Could you check a few things on this model? Use its own coordinates, in mm. A direction names the side the tool comes from. Round coordinates to 2 decimals unless told otherwise and drop trailing zeros. Write each loop counter-clockwise with the first axis right and the second up, starting at its lowest first coordinate (ties: lowest second). Pieces come first, ordered by that corner, then holes. Notation, with made-up numbers: M -28,20.5 L 8,20.5 A15 ccw 8,36.5 Z; hole C 44.25,70 d7. An arc over 180 degrees is marked long. One line per item, written item: value. Start each with the question number.
(1) I want a section at D-D on z = 0.5. Please give me the cut outline in (x, y), and give its area (4 significant figures).
(2) I want a section at C-C on x = -1. Please give me the cut outline in (y, z).
(3) I want a section at B-B on z = 5. Please give me the cut outline in (x, y).
(4) Which directions (+Z, -Z, +X, -X, +Y, -Y) give clear straight access to the entire face, cutting with the end or side of a thin tool? Please do faces 5 (the face through (-12, -12, 6)), 6 (the face through (5, 6, 1)), 7 (the face through (-9, -11, 4)).
(5) I want a section at A-A on y = -5.25. Please give me the cut outline in (x, z).
(6) Thinking about a two-plate mould opening in Z: for faces 1 (the face through (12, -12, 6)), 2 (the face through (-10, -13, 3)), 3 (the face through (-9.36, 11.99, 5.84)), 4 (the face through (8.9, -12, 5)), which applies, released by +Z, released by -Z, zero draft, split by the parting line, or undercut?
(7) I'm going to push flat-ended pins straight in: pin 1 Ø3 at (x, y) = (-5.5, 5) entering from +Z; pin 2 Ø2 at (x, z) = (-4.5, 2) entering from -Y; pin 3 Ø2.5 at (x, z) = (-2.5, 6) entering from -Y. Where does each tip first touch, or does it pass through?
(8) If I drill on L1, parallel to Y at x = 4.75, z = 1.75; L2, parallel to Z at x = -9.9, y = -11.7; L3, parallel to Y at x = 2, z = 5.5, over which ranges is the centre line in solid material (lowest first)?
```python
from build123d import *

# Parameters (mm, degrees)
F0_W        = 26
F0_H        = 2
F1_DEPTH    = 8
F0_W_2      = 6.25
F2_DEPTH    = 3
F3_T1_DEPTH = 27
F3_T3_DEPTH = 27
F4_R        = 1
F5_DEPTH    = 30


# Not quite as in the source:
# - a fillet or chamfer that OpenCascade refuses, or shapes differently, is made with other operations: its cross-section is extruded or revolved along the edge and cut away or added


with BuildPart() as f1:
    # F0 (on Top) → F1 (new body)
    with BuildSketch(Plane.XY):
        with Locations((0, 12)):
            Rectangle(F0_W, F0_H)
    extrude(amount=F1_DEPTH)



with BuildPart() as f1b:
    # F0 (on Top) → F1, piece 2 (new body)
    with BuildSketch(Plane.XY):
        with Locations((-9.875, -12)):
            Rectangle(F0_W_2, F0_H)
    extrude(amount=F1_DEPTH)


with BuildPart() as f1c:
    # F0 (on Top) → F1, piece 3 (new body)
    with BuildSketch(Plane.XY):
        with Locations((9.875, -12)):
            Rectangle(F0_W_2, F0_H)
    extrude(amount=F1_DEPTH)


with BuildPart() as f1_1:
    add(f1.part)

    add(f1b.part)  # F2 merges F1b

    add(f1c.part)  # F2 merges F1c
    # F0 (on Top) → F2 (join)
    with BuildSketch(Plane.XY):
        Polygon((6.75, -11), (13, -11), (13, 11), (-13, 11), (-13, -11), (-6.75, -11), (-6.75, 6), (-3.9725974202, 6), (-3.9725974202, 7), (4.0274025798, 7), (4.0274025798, 6), (6.75, 6), align=None)
    extrude(amount=F2_DEPTH)

    # F3: fillet of radius 5 on 6 edges, made by hand

    # F3_s2 → F3_t1 (cut)
    with BuildSketch(Plane.XZ.offset(-1.5)):
        with BuildLine():
            ThreePointArc((-8, 8), (-11.5355339059, 6.5355339059), (-13, 3))
            Line((-13, 3), (-13, 8))
            Line((-13, 8), (-8, 8))
        make_face()
        with BuildLine():
            ThreePointArc((-6.75, 3), (-8.2144660941, 6.5355339059), (-11.75, 8))
            Line((-11.75, 8), (-6.75, 8))
            Line((-6.75, 8), (-6.75, 3))
        make_face()
        with BuildLine():
            ThreePointArc((11.75, 8), (8.2144660941, 6.5355339059), (6.75, 3))
            Line((6.75, 3), (6.75, 8))
            Line((6.75, 8), (11.75, 8))
        make_face()
        with BuildLine():
            ThreePointArc((8, 8), (11.5355339059, 6.5355339059), (13, 3))
            Line((13, 3), (13, 8))
            Line((13, 8), (8, 8))
        make_face()
    extrude(amount=F3_T1_DEPTH, mode=Mode.SUBTRACT)

    # F3_s4 → F3_t3 (cut)
    with BuildSketch(Plane.XZ.offset(-25.5)):
        with BuildLine():
            ThreePointArc((8, 8), (11.5355339059, 6.5355339059), (13, 3))
            Line((13, 3), (13, 8))
            Line((13, 8), (8, 8))
        make_face()
        with BuildLine():
            ThreePointArc((-13, 3), (-11.5355339059, 6.5355339059), (-8, 8))
            Line((-8, 8), (-13, 8))
            Line((-13, 8), (-13, 3))
        make_face()
    extrude(amount=F3_T3_DEPTH, mode=Mode.SUBTRACT)

    # F4 (on face) → F5 (cut)
    with BuildSketch(Plane.XZ.offset(13)):
        with Locations((-9.9, 5)):
            Circle(F4_R)
        with Locations((9.9, 5)):
            Circle(F4_R)
    extrude(amount=-F5_DEPTH, mode=Mode.SUBTRACT)


solid = f1_1.part
```
Found:
1. outline: M -13,-13 L -6.75,-13 L -6.75,6 L -3.97,6 L -3.97,7 L 4.03,7 L 4.03,6 L 6.75,6 L 6.75,-13 L 13,-13 L 13,13 L -13,13 Z
1. area: 411.5 mm²
2. outline: M 7,0 L 13,0 L 13,8 L 11,8 L 11,3 L 7,3 Z
3. outline: M -12.58,-13 L -10.9,-13 L -10.9,-11 L -12.58,-11 Z; M -12.58,11 L -10.9,11 L -10.9,13 L -12.58,13 Z; M -8.9,-13 L -7.17,-13 L -7.17,-11 L -8.9,-11 Z; M -8.9,11 L 8.9,11 L 8.9,13 L -8.9,13 Z; M 7.17,-13 L 8.9,-13 L 8.9,-11 L 7.17,-11 Z; M 10.9,-13 L 12.58,-13 L 12.58,-11 L 10.9,-11 Z; M 10.9,11 L 12.58,11 L 12.58,13 L 10.9,13 Z
4. face 5: +Z, -X, +Y, -Y
4. face 6: +Z, -Z, -Y
4. face 7: +Z, +X, -X
5. outline: M -13,0 L -6.75,0 L -6.75,3 L -13,3 Z; M 6.75,0 L 13,0 L 13,3 L 6.75,3 Z
6. face 1: released by +Z
6. face 2: zero draft
6. face 3: undercut
6. face 4: undercut
7. pin 1: stops at z = 3
7. pin 2: stops at y = 6
7. pin 3: stops at y = 11
8. L1: y = 6 to 13
8. L2: z = 0 to 4, 6 to 7.62
8. L3: y = 11 to 13
